```python
from build123d import *

# Parameters (mm, degrees)
CROQUIS1_R                 = 9.525
CROQUIS1_R_2               = 9
SALIENTE_EXTRUIR1_DEPTH    = 115
CROQUIS2_R                 = 1.5875
CORTAR_EXTRUIR1_DEPTH      = 10.525
CORTAR_EXTRUIR1_DEPTH_BACK = 10.525
CROQUIS3_R                 = 1.5875
CORTAR_EXTRUIR2_DEPTH      = 10.5250001
CORTAR_EXTRUIR2_DEPTH_BACK = 10.5250001


with BuildPart() as part:
    # Croquis1 → Saliente-Extruir1 (new body)
    with BuildSketch(Plane.XY):
        Circle(CROQUIS1_R)
        Circle(CROQUIS1_R_2, mode=Mode.SUBTRACT)
    extrude(amount=SALIENTE_EXTRUIR1_DEPTH)

    # Croquis2 → Cortar-Extruir1 (cut, two sides)
    with BuildSketch(Plane(origin=(0, 0, 0), x_dir=(0, 0, -1), z_dir=(1, 0, 0))) as cortar_extruir1_sk:
        with Locations((-9.8, 0)):
            Circle(CROQUIS2_R)
    extrude(amount=CORTAR_EXTRUIR1_DEPTH, mode=Mode.SUBTRACT)
    extrude(cortar_extruir1_sk.sketch, amount=-CORTAR_EXTRUIR1_DEPTH_BACK, mode=Mode.SUBTRACT)

    # Croquis3 → Cortar-Extruir2 (cut, two sides)
    with BuildSketch(Plane(origin=(0, 0, 0), x_dir=(1, 0, 0), z_dir=(0, 1, 0))) as cortar_extruir2_sk:
        with Locations((0, -107.0025)):
            Circle(CROQUIS3_R)
    extrude(amount=CORTAR_EXTRUIR2_DEPTH, mode=Mode.SUBTRACT)
    extrude(cortar_extruir2_sk.sketch, amount=-CORTAR_EXTRUIR2_DEPTH_BACK, mode=Mode.SUBTRACT)


solid = part.part
```
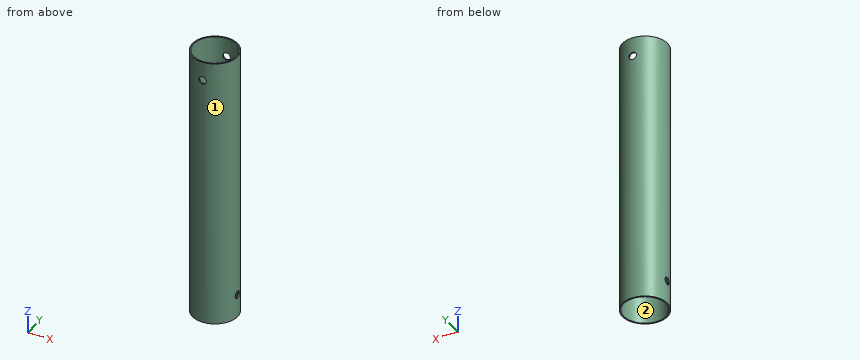
Could you check a few things on this model? Use its own coordinates, in mm. Face numbers are marked on the shaded views. Round coordinates to 2 decimals unless told otherwise and drop trailing zeros. Loops run counter-clockwise (first coordinate to the right, second up) from the corner with the lowest first, then second, coordinate; pieces in that order, holes last. Notation, with made-up numbers: (7.5, -2) - (47.5, -2) arc R24 ccw to (47.5, 20) - close; hole circle Ø7 at (20, 45.5). An arc over 180 degrees is marked (long way). Answer in a Markdown table with one row per item. Add a question column.
(1) If we section it at C-C (y = -4.25): Please give me the cut outline in (x, z).
(2) I'm going to push flat-ended pins straight in: pin 1 (6 mm diameter, centred on x = 4.5, z = 28, fed in from +Y); pin 2 (3 mm diameter, centred on y = -3.5, z = 27, fed in from +X); pin 3 (1.5 mm diameter, centred on x = 1.5, z = 80, fed in from +Y). Where does each tip first touch, or does it pass through?
(3) If we mould it in two halves opening along Y, with no side actions, what happens to the marked faces 1 and 2? For each: pulls with the +Y half, pulls with the -Y half, needs draft (parallel to the pull), parting line crosses it, or undercut.
(4) If we section it at B-B (x = 0): Please give me the cut outline in (y, z) (3 decimals), plus the area to 3 significant figures.
(5) If we section it at A-A (y = 0): Please give me the cut outline in (x, z) (1 decimal), plus the area to 3 significant figures.
(6) I need wall thicknesses on line 1 along Z through (x, y) = (0, -9.3) (3 decimals); line 2 along X through (y, z) = (0, 42) (3 decimals); line 3 along X through (y, z) = (6.25, 61). Which ranges of each line are inside material? Lowest first, please.
(7) If we section it at D-D (z = 101.5): Please give me the cut outline in (x, y) (3 decimals), plus the area to 3 significant figures.
Model answer:
| question | item | result |
|---|---|---|
| 1 | outline | (-8.52, 0) - (-7.93, 0) - (-7.93, 115) - (-8.52, 115) - close; (7.93, 0) - (8.52, 0) - (8.52, 115) - (7.93, 115) - close |
| 2 | pin 1 | stops at y = 9.41 |
| 2 | pin 2 | stops at x = 9.31 |
| 2 | pin 3 | stops at y = 9.5 |
| 3 | face 1 | parting line crosses it |
| 3 | face 2 | undercut |
| 4 | outline | (-9.525, 0) - (-9, 0) - (-9, 105.415) - (-9.525, 105.415) - close; (-9.525, 108.59) - (-9, 108.59) - (-9, 115) - (-9.525, 115) - close; (9, 0) - (9.525, 0) - (9.525, 105.415) - (9, 105.415) - close; (9, 108.59) - (9.525, 108.59) - (9.525, 115) - (9, 115) - close |
| 4 | area | 117 mm² |
| 5 | outline | (-9.5, 0) - (-9, 0) - (-9, 8.2) - (-9.5, 8.2) - close; (-9.5, 11.4) - (-9, 11.4) - (-9, 115) - (-9.5, 115) - close; (9, 0) - (9.5, 0) - (9.5, 8.2) - (9, 8.2) - close; (9, 11.4) - (9.5, 11.4) - (9.5, 115) - (9, 115) - close |
| 5 | area | 117 mm² |
| 6 | line 1 | z = 0 to 105.415, 108.59 to 115 |
| 6 | line 2 | x = -9.525 to -9, 9 to 9.525 |
| 6 | line 3 | x = -7.19 to -6.48, 6.48 to 7.19 |
| 7 | outline | circle Ø19.05 at (0, 0); hole circle Ø18 at (0, 0) |
| 7 | area | 30.6 mm² |
